Design review of the part built by this model. Coordinates are the model's own, in mm. A direction names the side the tool comes from. Coordinates: 2 decimals unless noted, no trailing zeros. Loops run counter-clockwise (first coordinate to the right, second up) from the corner with the lowest first, then second, coordinate; pieces in that order, holes last. Notation, with made-up numbers: (50.25, -36) -> (80.25, -36) arc R29 cw to (80.25, 0) -> close; hole circle Ø3 at (53, 33). An arc over 180 degrees is marked (long way). Answer as a JSON object with one key per item and string values.
```python
from build123d import *

# Parameters (mm, degrees)
IZIM1_W                     = 110
IZIM1_H                     = 87
Y_KSEKLIK_EKSTR_ZYON1_DEPTH = 3
RADYUS1_R                   = 2
IZIM2_R                     = 4
Y_KSEKLIK_EKSTR_ZYON2_DEPTH = 27
IZIM4_R                     = 6.5
KES_EKSTR_ZYON1_DEPTH       = 13
IZIM5_R                     = 1.5
KES_EKSTR_ZYON2_DEPTH       = 10


with BuildPart() as part:
    # Çizim1 → Yükseklik-Ekstrüzyon1 (new body)
    with BuildSketch(Plane(origin=(0, 0, 0), x_dir=(1, 0, 0), z_dir=(0, 1, 0))):
        Rectangle(IZIM1_W, IZIM1_H)
    extrude(amount=Y_KSEKLIK_EKSTR_ZYON1_DEPTH)

    # Radyus1
    radyus1_edges = [part.edges().sort_by_distance(p)[0] for p in [
        (55, 1.5, 43.5),
        (-55, 1.5, 43.5),
        (-55, 1.5, -43.5),
        (55, 1.5, -43.5),
    ]]
    fillet(radyus1_edges, radius=RADYUS1_R)

    # Çizim2 → Yükseklik-Ekstrüzyon2 (add)
    with BuildSketch(Plane(origin=(0, 3, 0), x_dir=(1, 0, 0), z_dir=(0, 1, 0))):
        with Locations(Location((-49, 37.5, 0), (0, 0, 90))):
            Circle(IZIM2_R)
        with Locations(Location((49, 37.5, 0), (0, 0, 90))):
            Circle(IZIM2_R)
        with Locations(Location((49, -37.5, 0), (0, 0, 90))):
            Circle(IZIM2_R)
        with Locations(Location((-49, -37.5, 0), (0, 0, 90))):
            Circle(IZIM2_R)
    extrude(amount=Y_KSEKLIK_EKSTR_ZYON2_DEPTH)

    # Çizim4 → Kes-Ekstrüzyon1 (cut)
    with BuildSketch(Plane.XZ):
        with Locations(Location((0, 33.5, 0), (0, 0, 270))):
            Circle(IZIM4_R)
    extrude(amount=-KES_EKSTR_ZYON1_DEPTH, mode=Mode.SUBTRACT)

    # Çizim5 → Kes-Ekstrüzyon2 (cut)
    with BuildSketch(Plane(origin=(0, 0, 0), x_dir=(-1, 0, 0), z_dir=(0, -1, 0))):
        with Locations(Location((-22.32, -22.43, 0), (0, 0, 90))):
            Circle(IZIM5_R)
        with Locations(Location((10.36, -21.88, 0), (0, 0, 90))):
            Circle(IZIM5_R)
        with Locations(Location((-24.94, 36.07, 0), (0, 0, 90))):
            Circle(IZIM5_R)
        with Locations(Location((24.72, 32.33, 0), (0, 0, 90))):
            Circle(IZIM5_R)
    extrude(amount=-KES_EKSTR_ZYON2_DEPTH, mode=Mode.SUBTRACT)


solid = part.part
```
1) Add section C-C, the plane y = 14. Give the boundary of the cut face in (x, z), and give its area (3 significant figures).
Completed:
{"outline": "circle Ø8 at (-49, -37.5); circle Ø8 at (-49, 37.5); circle Ø8 at (49, -37.5); circle Ø8 at (49, 37.5)", "area": "201 mm²"}
2) Add section A-A, the plane z = -32.33. Give the boundary of the cut face in (x, y).
Completed:
{"outline": "(-55, 0) -> (-26.22, 0) -> (-26.22, 3) -> (-55, 3) -> close; (-23.22, 0) -> (55, 0) -> (55, 3) -> (-23.22, 3) -> close"}
3) Wall thickness on probe 1 along X at (y, z) = (2, -32.33); probe 2 along X at (y, z) = (0.8, 33.5); probe 3 along X at (y, z) = (2.1, 21.88): over which ranges is each line inside the solid? List them lowest first.
Completed:
{"probe 1": "-55 to -26.22, -23.22 to 55", "probe 2": "-55 to -6.5, 6.5 to 55", "probe 3": "-55 to -11.86, -8.86 to 20.92, 23.72 to 55"}
4) Add section B-B, the plane x = -49. Give the boundary of the cut face in (y, z).
Completed:
{"outline": "(0, -43.5) -> (3, -43.5) -> (3, -41.5) -> (30, -41.5) -> (30, -33.5) -> (3, -33.5) -> (3, 33.5) -> (30, 33.5) -> (30, 41.5) -> (3, 41.5) -> (3, 43.5) -> (0, 43.5) -> close"}
5) Add section D-D, the plane z = -13.5. Give the boundary of the cut face in (x, y).
Completed:
{"outline": "(-55, 0) -> (55, 0) -> (55, 3) -> (-55, 3) -> close"}
6) The part is to be moulded in two halves that separate along Z. For faces 1 (the flat face through (-1, 1, 43.5)), 2 (the cylindrical face through (-10.935, 1.479, 20.494)), 3 (the flat face through (55, 1, 1)), say which applies: pulls with the +Z half, pulls with the -Z half, needs draft (parallel to the pull), parting line crosses it, or undercut.
Completed:
{"face 1": "pulls with the +Z half", "face 2": "undercut", "face 3": "needs draft"}
7) Clearance check with flat-ended pins moving along their axes: pin 1 Ø4 at (x, z) = (22.32, 22.43) entering from +Y; pin 2 Ø2.5 at (x, z) = (-24.72, -32.33) entering from -Y. State where each tip first meets the part, or that it passes through.
Completed:
{"pin 1": "y = 3", "pin 2": "through"}
8) For faces 4 (the flat face through (-49, 30, -37)), 5 (the cylindrical face through (-46.6, 16.3, -34.3)), list the 3-axis set-ups (+Z, -Z, +X, -X, +Y, -Y) from which the entire face can be reached by the end or side of a thin tool; tool diameter is ignored.
Completed:
{"face 4": "+Z, -Z, +X, -X, +Y", "face 5": "+Y"}
